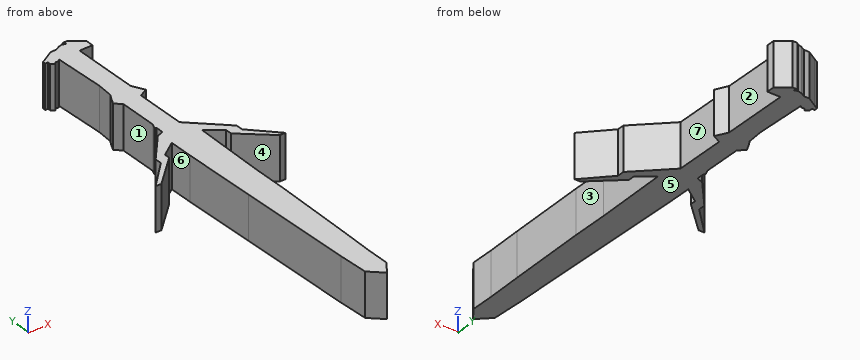
```python
from build123d import *

# Parameters (mm, degrees)
F1_DEPTH = 12.7


with BuildPart() as f1:
    # F0 (on Top) → F1 (new body)
    with BuildSketch(Plane.XY):
        Polygon((8.4674097598, 56.3226677477), (4.9993731081, 59.1430924833), (3.5796526354, 59.105347842), (4.0142790642, 58.5837887803), (3.9040301926, 58.2936815917), (3.0076738913, 58.6343221366), (1.81281392, 58.3214089274), (0.4375161952, 57.63842538), (0, 57.63842538), (-1.0647438467, 57.63842538), (-3.7269797176, 56.0346469283), (-5.1362086087, 55.2338398993), (-5.1362086087, 54.3800778687), (-4.324192436, 54.3800778687), (-4.324192436, 53.5804792602), (-3.2959955279, 52.7911260724), (-2.8494205326, 53.3728264272), (-1.9739218988, 53.3728264272), (-1.4901272083, 53.7990161207), (-1.4361526119, 51.9273541868), (-1.0647438467, 39.0481166542), (-1.4684260823, 34.2683680356), (-2.1647270769, 33.138576895), (-3.2786394004, 30.8706443757), (-1.5108085936, 29.2773563415), (-1.5108085936, 18.0350095034), (-2.0992092323, 16.6827999055), (-1.7486788565, 16.2351131439), (-1.7486788565, 14.0109397471), (-3.6478310358, 13.3241694421), (-10.2832335979, 5.4679820314), (-10.2832335979, 3.4643800464), (-17.465846613, -3.8865045644), (-15.7476849854, -3.8865045644), (-7.3585305363, 4.1265715845), (-7.3585305363, 5.7251015678), (-2.9132614987, 8.9498246089), (-2.9132614987, 2.0007098744), (-2.5243267883, -19.7883937508), (-1.9065504894, -54.3977804482), (-1.5426465543, -63.1300359964), (2.1701699588, -66.6309818625), (4.7807293013, -62.9719868302), (4.7807293013, -56.274600327), (5.0807259977, -46.0444651544), (5.579222925, -22.7906536311), (5.579222925, -12.2377127409), (6.0616787523, 9.1150859371), (10.5058038607, 5.7430174202), (10.5058038607, 3.8492596457), (19.0487038344, -3.5993366037), (20.6745713949, -3.5993366037), (13.642212376, 3.7180308718), (13.642212376, 5.8058663271), (4.0112765072, 15.0460293517), (4.0112765072, 29.7966579315), (6.4584943466, 31.0973599553), (4.653096199, 34.4941429794), (4.653096199, 50.1591525972), (4.653096199, 54.0697947145), (8.4674097598, 54.0697947145), align=None)
    extrude(amount=F1_DEPTH)


solid = f1.part
```
The model under review builds one solid part; all positions refer to its coordinate system, in mm. Face numbers are marked on the shaded views. A direction names the side the tool comes from. Round coordinates to 2 decimals unless told otherwise and drop trailing zeros. Loops run counter-clockwise (first coordinate to the right, second up) from the corner with the lowest first, then second, coordinate; pieces in that order, holes last. Notation, with made-up numbers: M 71.5,74.5 L 94.5,74.5 A14 ccw 94.5,97.5 Z; hole C -14,77 d2. An arc over 180 degrees is marked long. Answer as a JSON object with one key per item and string values.
(1) To check wall thickness, follow line 1 along X through (y, z) = (6.5, 8); line 2 along Y through (x, z) = (-4, 10.75); line 3 along X through (y, z) = (16.5, 9). State the ranges of each line that lie inside material, in increasing order.
Resolved:
{"line 1": "-9.41 to -6.29, -2.91 to 6, 9.51 to 12.92", "line 2": "8.16 to 12.91, 53.33 to 55.88", "line 3": "-1.96 to 4.01"}
(2) Tool access review of the marked faces 1, 2, 3 and 4: name each direction out of +Z, -Z, +X, -X, +Y, -Y from which nothing blocks a thin tool from reaching the whole face with its end or side.
Resolved:
{"face 1": "+Z, -Z, -X", "face 2": "+Z, -Z, +X", "face 3": "+Z, -Z, +X, -Y", "face 4": "+Z, -Z, -Y"}
(3) Draft analysis for pull direction X (two halves, no side actions). For the marked faces 5, 6 and 7, state which applies: released by +X, released by -X, zero draft, split by the parting line, or undercut.
Resolved:
{"face 5": "zero draft", "face 6": "undercut", "face 7": "released by +X"}
(4) Take a section at B-B on x = -14. Give the boundary of the cut face in (y, z), and give its area (3 significant figures).
Resolved:
{"outline": "M -2.22,0 L -0.34,0 L -0.34,12.7 L -2.22,12.7 Z", "area": "23.8 mm²"}
(5) Take a section at A-A on y = 21.5. Give the boundary of the cut face in (x, z), and give its area (3 significant figures).
Resolved:
{"outline": "M -1.51,0 L 4.01,0 L 4.01,12.7 L -1.51,12.7 Z", "area": "70.1 mm²"}
(6) Clearance check with flat-ended pins moving along their axes: P1, Ø4, axis at y = 15, z = 6, coming from the +X side; P2, Ø0.7, axis at y = 55.5, z = 5, coming from the +X side; P3, Ø1, axis at x = 16, z = 7, coming from the -Y side; P4, Ø6, axis at x = -5, y = -40, coming from the +Z side. State where each tip first meets the part, or that it passes through.
Resolved:
{"P1": "x = 6.14", "P2": "x = 8.47", "P3": "y = -1.38", "P4": "z = 12.7"}
